Read the model definition and answer for the solid it produces. Units are mm, in the model's axes. A direction names the side the tool comes from. Give positions to 0.01 mm unless a question says otherwise; leave off trailing zeros. Order: outer loops, then holes, each group sorted by start corner. A loop starts at its lowest first (then second) coordinate and runs counter-clockwise, first axis right, second up. Notation, with made-up numbers: (9, 88.5) -> (46, 88.5) arc R10 cw to (46, 99.5) -> close; hole circle Ø11 at (-38.75, -13). An arc over 180 degrees is marked (long way). One line per question, with ' | ' between items. Start each with the question number.
```python
from build123d import *

# Parameters (mm, degrees)
SKETCH013_AS_DRAWN_W                      = 11.85
SKETCH013_AS_DRAWN_H                      = 8.5
EXTRUDE018_DEPTH                          = 2
EXTRUDE018_ONTO_SKETCH013_ROLL_ANGLE      = 90
SKETCH009_AS_DRAWN_W                      = 11.85
SKETCH009_AS_DRAWN_H                      = 8.5
EXTRUDE017_DEPTH                          = 10
EXTRUDE017_ONTO_SKETCH009_ROLL_ANGLE      = 90
SKETCH012_AS_DRAWN_W                      = 14.5
SKETCH012_AS_DRAWN_H                      = 14.25
EXTRUDE016_DEPTH                          = 10
EXTRUDE016_ONTO_SKETCH012_ROLL_ANGLE      = 90
SKETCH010_AS_DRAWN_W                      = 9
SKETCH010_AS_DRAWN_H                      = 4
EXTRUDE015_DEPTH                          = 30
EXTRUDE015_ONTO_SKETCH010_ROLL_ANGLE      = 90
SKETCH011_AS_DRAWN_W                      = 11.5
SKETCH011_AS_DRAWN_H                      = 5
EXTRUDE014_DEPTH                          = 8
EXTRUDE014_ONTO_SKETCH011_ROLL_ANGLE      = 90
EXTRUDE013_DEPTH                          = 20
SKETCH006_AS_DRAWN_W                      = 3
SKETCH006_AS_DRAWN_H                      = 2
EXTRUDE011_DEPTH                          = 3
EXTRUDE011_ONTO_SKETCH006_ROLL_ANGLE      = 90
EXTRUDE011_ONTO_SKETCH006_PLACEMENT_ANGLE = 180
EXTRUDE010_DEPTH                          = 4
EXTRUDE008_DEPTH                          = 16
EXTRUDE008_ONTO_SKETCH004_ROLL_ANGLE      = 90
EXTRUDE008_ONTO_SKETCH004_PLACEMENT_ANGLE = 180
EXTRUDE002_DEPTH                          = 1.25
EXTRUDE_DEPTH                             = 4
EXTRUDE004_DEPTH                          = 18.25
EXTRUDE012_DEPTH                          = 9
FILLET_R                                  = 1
FILLET001_R                               = 1
FILLET002_R                               = 2
FILLET003_R                               = 2
FILLET004_R                               = 1
FILLET005_R                               = 2
FILLET006_R                               = 1


with BuildPart() as extrude018:
    # Sketch013 as drawn → Extrude018 (new)
    with BuildSketch(Plane.XY):
        Rectangle(SKETCH013_AS_DRAWN_W, SKETCH013_AS_DRAWN_H)
    extrude(amount=-EXTRUDE018_DEPTH)


with BuildPart() as extrude018_1:
    # Extrude018 onto Sketch013 roll: moved
    add(extrude018.part.rotate(Axis((0, 0, 0), (1, 0, 0)), EXTRUDE018_ONTO_SKETCH013_ROLL_ANGLE))


with BuildPart() as extrude018_2:
    # Extrude018 onto Sketch013 placement: moved
    add(extrude018_1.part.moved(Location((0, -28, 0))))


with BuildPart() as extrude017:
    # Sketch009 as drawn → Extrude017 (new)
    with BuildSketch(Plane.XY):
        Rectangle(SKETCH009_AS_DRAWN_W, SKETCH009_AS_DRAWN_H)
    extrude(amount=EXTRUDE017_DEPTH)


with BuildPart() as extrude017_1:
    # Extrude017 onto Sketch009 roll: moved
    add(extrude017.part.rotate(Axis((0, 0, 0), (1, 0, 0)), EXTRUDE017_ONTO_SKETCH009_ROLL_ANGLE))


with BuildPart() as extrude017_2:
    # Extrude017 onto Sketch009 placement: moved
    add(extrude017_1.part.moved(Location((0, -26, 0))))


with BuildPart() as cut006:
    # Sketch012 as drawn → Extrude016 (new)
    with BuildSketch(Plane.XY):
        with Locations((0, -1.875)):
            Rectangle(SKETCH012_AS_DRAWN_W, SKETCH012_AS_DRAWN_H)
    extrude(amount=EXTRUDE016_DEPTH)


with BuildPart() as cut006_1:
    # Extrude016 onto Sketch012 roll: moved
    add(cut006.part.rotate(Axis((0, 0, 0), (1, 0, 0)), EXTRUDE016_ONTO_SKETCH012_ROLL_ANGLE))


with BuildPart() as cut006_2:
    # Extrude016 onto Sketch012 placement: moved
    add(cut006_1.part.moved(Location((0, -26, 0))))

    # Cut006: cut Extrude017
    add(extrude017_2.part, mode=Mode.SUBTRACT)


with BuildPart() as extrude015:
    # Sketch010 as drawn → Extrude015 (new)
    with BuildSketch(Plane.XY):
        Rectangle(SKETCH010_AS_DRAWN_W, SKETCH010_AS_DRAWN_H)
    extrude(amount=EXTRUDE015_DEPTH)


with BuildPart() as extrude015_1:
    # Extrude015 onto Sketch010 roll: moved
    add(extrude015.part.rotate(Axis((0, 0, 0), (1, 0, 0)), EXTRUDE015_ONTO_SKETCH010_ROLL_ANGLE))


with BuildPart() as extrude015_2:
    # Extrude015 onto Sketch010 placement: moved
    add(extrude015_1.part)


with BuildPart() as extrude014:
    # Sketch011 as drawn → Extrude014 (new)
    with BuildSketch(Plane.XY):
        with Locations((0, -0.5)):
            Rectangle(SKETCH011_AS_DRAWN_W, SKETCH011_AS_DRAWN_H)
    extrude(amount=EXTRUDE014_DEPTH)


with BuildPart() as extrude014_1:
    # Extrude014 onto Sketch011 roll: moved
    add(extrude014.part.rotate(Axis((0, 0, 0), (1, 0, 0)), EXTRUDE014_ONTO_SKETCH011_ROLL_ANGLE))


with BuildPart() as extrude014_2:
    # Extrude014 onto Sketch011 placement: moved
    add(extrude014_1.part.moved(Location((0, -18, 0))))


with BuildPart() as extrude013:
    # Sketch008 → Extrude013 (new body)
    with BuildSketch(Plane.XY):
        with BuildLine():
            ThreePointArc((-19.054199, -15), (0, -24.25), (19.054199, -15))
            Line((-19.054199, -15), (19.054199, -15))
        make_face()
    extrude(amount=EXTRUDE013_DEPTH)


with BuildPart() as extrude011:
    # Sketch006 as drawn → Extrude011 (new)
    with BuildSketch(Plane.XY):
        with Locations((26.45538, 9.53866)):
            Rectangle(SKETCH006_AS_DRAWN_W, SKETCH006_AS_DRAWN_H)
    extrude(amount=-EXTRUDE011_DEPTH)


with BuildPart() as extrude011_1:
    # Extrude011 onto Sketch006 roll: moved
    add(extrude011.part.rotate(Axis((0, 0, 0), (1, 0, 0)), EXTRUDE011_ONTO_SKETCH006_ROLL_ANGLE))


with BuildPart() as extrude011_2:
    # Extrude011 onto Sketch006 placement: moved
    add(extrude011_1.part.rotate(Axis((0, 0, 0), (0, 0, 1)), EXTRUDE011_ONTO_SKETCH006_PLACEMENT_ANGLE))


with BuildPart() as extrude010:
    # Sketch005 → Extrude010 (new body)
    with BuildSketch(Plane.XY.offset(18.25)):
        with BuildLine():
            ThreePointArc((-30, 0), (0, -30), (30, 0))
            Line((22.5, 0), (30, 0))
            Line((22.5, -17), (22.5, 0))
            Line((-22.5, -17), (22.5, -17))
            Line((-22.5, 0), (-22.5, -17))
            Line((-30, 0), (-22.5, 0))
        make_face()
    extrude(amount=-EXTRUDE010_DEPTH)


with BuildPart() as extrude008:
    # Sketch004 as drawn → Extrude008 (new)
    with BuildSketch(Plane.XY):
        Polygon((-22.75, 4), (22.75, 4), (22.75, 6), (25.75, 6), (25.75, 12.75), (19.5, 12.75), (19.5, 14.75), (20.5, 14.75), (20.5, 16.75), (19.5, 16.75), (19.5, 18.25), (-19.5, 18.25), (-19.5, 16.75), (-20.5, 16.75), (-20.5, 14.75), (-19.5, 14.75), (-19.5, 12.75), (-25.75, 12.75), (-25.75, 6), (-22.75, 6), align=None)
    extrude(amount=-EXTRUDE008_DEPTH)


with BuildPart() as extrude008_1:
    # Extrude008 onto Sketch004 roll: moved
    add(extrude008.part.rotate(Axis((0, 0, 0), (1, 0, 0)), EXTRUDE008_ONTO_SKETCH004_ROLL_ANGLE))


with BuildPart() as extrude008_2:
    # Extrude008 onto Sketch004 placement: moved
    add(extrude008_1.part.rotate(Axis((0, 0, 0), (0, 0, 1)), EXTRUDE008_ONTO_SKETCH004_PLACEMENT_ANGLE))


with BuildPart() as extrude002:
    # Sketch003 → Extrude002 (new body)
    with BuildSketch(Plane.XY.offset(2)):
        with BuildLine():
            ThreePointArc((-25.25, 0), (0, -25.25), (25.25, 0))
            Line((-25.25, 0), (25.25, 0))
        make_face()
    extrude(amount=EXTRUDE002_DEPTH)


with BuildPart() as obj1:
    # Sketch002 → Extrude (new body)
    with BuildSketch(Plane.XY):
        with BuildLine():
            ThreePointArc((-24.25, 0), (0, -24.25), (24.25, 0))
            Line((-24.25, 0), (24.25, 0))
        make_face()
    extrude(amount=EXTRUDE_DEPTH)

    # Fusion: union Extrude002
    add(extrude002.part)


with BuildPart() as cut003:
    # Sketch001 → Extrude004 (new body)
    with BuildSketch(Plane.XY):
        with BuildLine():
            ThreePointArc((-27.5, 0), (0, -27.5), (27.5, 0))
            Line((-27.5, 0), (27.5, 0))
        make_face()
    extrude(amount=EXTRUDE004_DEPTH)

    # Cut: cut obj1
    add(obj1.part, mode=Mode.SUBTRACT)

    # Cut001: cut Extrude008
    add(extrude008_2.part, mode=Mode.SUBTRACT)

    # Cut002: cut Extrude010
    add(extrude010.part, mode=Mode.SUBTRACT)

    # Cut003: cut Extrude011
    add(extrude011_2.part, mode=Mode.SUBTRACT)


with BuildPart() as fillet006:
    # Sketch007 → Extrude012 (new body)
    with BuildSketch(Plane.XY):
        with BuildLine():
            ThreePointArc((-27.5, 0), (0, -27.5), (27.5, 0))
            Line((24.25, 0), (27.5, 0))
            ThreePointArc((-24.25, 0), (0, -24.25), (24.25, 0))
            Line((-27.5, 0), (-24.25, 0))
        make_face()
    extrude(amount=-EXTRUDE012_DEPTH)

    # Fusion001: union Cut003
    add(cut003.part)

    # Cut004: cut Extrude013
    add(extrude013.part, mode=Mode.SUBTRACT)

    # Fillet
    fillet_edges = [fillet006.edges().sort_by_distance(p)[0] for p in [
        (-19.454695, -17, 14.25),
        (19.454695, -17, 14.25),
    ]]
    fillet(fillet_edges, radius=FILLET_R)

    # Fillet001
    fillet001_edges = [fillet006.edges().sort_by_distance(p)[0] for p in [
        (-22.5, -7.905694, 14.25),
        (22.5, -7.905694, 14.25),
    ]]
    fillet(fillet001_edges, radius=FILLET001_R)

    # Fillet002
    fillet002_edges = [fillet006.edges().sort_by_distance(p)[0] for p in [
        (25.75, -4.826684, 12.75),
    ]]
    fillet(fillet002_edges, radius=FILLET002_R)

    # Fillet003
    fillet003_edges = [fillet006.edges().sort_by_distance(p)[0] for p in [
        (-25.75, -4.826684, 12.75),
    ]]
    fillet(fillet003_edges, radius=FILLET003_R)

    # Fusion002: union Extrude014
    add(extrude014_2.part)

    # Cut005: cut Extrude015
    add(extrude015_2.part, mode=Mode.SUBTRACT)

    # Fusion003: union Cut006
    add(cut006_2.part)

    # Cut007: cut Extrude018
    add(extrude018_2.part, mode=Mode.SUBTRACT)

    # Fillet004
    fillet004_edges = [fillet006.edges().sort_by_distance(p)[0] for p in [
        (4.5, -22, -2),
        (-4.5, -22, -2),
    ]]
    fillet(fillet004_edges, radius=FILLET004_R)

    # Fillet005
    fillet005_edges = [fillet006.edges().sort_by_distance(p)[0] for p in [
        (0, -24.25, -3),
    ]]
    fillet(fillet005_edges, radius=FILLET005_R)

    # Fillet006
    fillet006_edges = [fillet006.edges().sort_by_distance(p)[0] for p in [
        (5.925, -32, 4.25),
        (-5.925, -32, 4.25),
    ]]
    fillet(fillet006_edges, radius=FILLET006_R)


solid = fillet006.part
```
Q1. Given P1, Ø1.1, axis at x = 20, y = -5.5, coming from the -Z side; P2, Ø6, axis at y = -31, z = 0, coming from the +X side; P3, Ø0.9, axis at y = -21.5, z = 1, coming from the -X side, each flat-ended and moving along its own axis, determine where each tip first touches the part or whether it passes through.
Q2. A cutting plane is placed at A-A, the plane z = 0.75. Determine the outline of the cut face in (x, y) (3 decimals).
Q3. A cutting plane is placed at D-D, the plane x = 13. Determine the outline of the cut face in (y, z), then the cut area to 3 significant figures.
Q4. Determine the mould class of faces 6 (the flat face through (23, -3, 4)), 7 (the flat face through (0, -25, 3.25)), 8 (the flat face through (-19, -17, 17)) for opening direction Z: pulls with the +Z half, pulls with the -Z half, needs draft (parallel to the pull), parting line crosses it, or undercut.
Q5. A cutting plane is placed at C-C, the plane y = -20.5. Determine the outline of the cut face in (x, z), then the cut area to 3 significant figures.
Q6. Find the intervals of material crossed by line 1 (Y direction, x = 16, z = 11.25); line 2 (X direction, y = -3, z = 0); line 3 (X direction, y = -11, z = 1.25), in increasing order.
Q7. Which of the six approach directions +Z, -Z, +X, -X, +Y, -Y give full straight-line access (tool end or side, diameter ignored) to faces 1 (the cylindrical face through (25.18, -5.49, 12.15)), 2 (the flat face through (-20.5, -8, 16)), 3 (the cylindrical face through (-0.533, -24.244, -6.021)), 4 (the flat face through (0, -31, -4.25)), 5 (the flat face through (0, -25, 14.25))?
Q8. A cutting plane is placed at B-B, the plane x = 0. Determine the outline of the cut face in (y, z), then the cut area to 3 significant figures.
Geometry results:
1) P1: z = 12.75 | P2: x = 7.25 | P3: x = -17.7
2) outline: (-27.5, 0) arc R27.5 ccw to (-7.25, -26.527) -> (-7.25, -36) -> (-5.925, -36) -> (-5.925, -26) -> (-4.5, -26) -> (-4.5, -18) -> (-5.75, -18) -> (-5.75, -23.558) arc R24.25 cw to (-24.25, 0) -> close; (4.5, -26) -> (5.925, -26) -> (5.925, -36) -> (7.25, -36) -> (7.25, -26.527) arc R27.5 ccw to (27.5, 0) -> (24.25, 0) arc R24.25 cw to (5.75, -23.558) -> (5.75, -18) -> (4.5, -18) -> close
3) outline: (-24.23, -9) -> (-20.47, -9) -> (-20.47, 2) -> (-21.65, 2) -> (-21.65, 3.25) -> (-20.47, 3.25) -> (-20.47, 14.25) -> (-24.23, 14.25) -> close | area: 86.0 mm²
4) face 6: pulls with the -Z half | face 7: undercut | face 8: needs draft
5) outline: (-18.33, -9) -> (-12.95, -9) -> (-12.95, 2) -> (-14.74, 2) -> (-14.74, 3.25) -> (-12.95, 3.25) -> (-12.95, 14.25) -> (-18.33, 14.25) -> close; (-5.75, -3) -> (5.75, -3) -> (5.75, 2) -> (4.5, 2) -> (4.5, -1) arc R1 cw to (3.5, -2) -> (-3.5, -2) arc R1 cw to (-4.5, -1) -> (-4.5, 2) -> (-5.75, 2) -> close; (12.95, -9) -> (18.33, -9) -> (18.33, 14.25) -> (12.95, 14.25) -> (12.95, 3.25) -> (14.74, 3.25) -> (14.74, 2) -> (12.95, 2) -> close | area: 267 mm²
6) line 1: -22.37 to -18.22 | line 2: -27.34 to -24.06, 24.06 to 27.34 | line 3: -25.2 to -21.61, 21.61 to 25.2
7) face 1: +Y, -Y | face 2: +Y | face 3: -Z, +Y | face 4: -Y | face 5: +Z, +X, -X, -Y
8) outline: (-36, -9) -> (-24.25, -9) -> (-24.25, -5) arc R2 cw to (-22.25, -3) -> (-18, -3) -> (-18, -2) -> (-26, -2) -> (-26, -4.25) -> (-36, -4.25) -> close; (-36, 4.25) -> (-26, 4.25) -> (-26, 2) -> (-25.25, 2) -> (-25.25, 3.25) -> (-24.25, 3.25) -> (-24.25, 14.25) -> (-27.5, 14.25) -> (-27.5, 5.25) -> (-36, 5.25) -> close | area: 111 mm²
